Work out the finished part from the listing and answer in its coordinate system (mm). A direction names the side the tool comes from. Round coordinates to 2 decimals unless told otherwise and drop trailing zeros. Order: outer loops, then holes, each group sorted by start corner. A loop starts at its lowest first (then second) coordinate and runs counter-clockwise, first axis right, second up. Notation, with made-up numbers: (24.5, 38) - (68.5, 38) arc R10 ccw to (68.5, 53) - close; hole circle Ø7 at (35, 72.5). An arc over 180 degrees is marked (long way). Put each result on its own line as item: value.
```python
from build123d import *

# Parameters (mm, degrees)
BOSS_EXTRUDE1_DEPTH        = 4
BOSS_EXTRUDE2_REACH        = 34.985
F_2_CLEARANCE_HOLE1_D      = 2.5
F_12_CLEARANCE_HOLE1_D     = 6
F_4_CLEARANCE_HOLE1_REACH  = 43.113
F_4_CLEARANCE_HOLE1_BORE_R = 1.65
SKETCH9_W                  = 1.65
SKETCH9_H                  = 32
FILLET1_R                  = 2


with BuildPart() as part:
    # Sketch1 → Boss-Extrude1 (new body)
    with BuildSketch(Plane(origin=(0, 0, 12), x_dir=(-1, 0, 0), z_dir=(0, 0, -1))):
        with BuildLine():
            Line((-17.88854382, -16), (17.88854382, -16))
            ThreePointArc((17.88854382, -16), (24, 0), (17.88854382, 16))
            Line((17.88854382, 16), (-17.88854382, 16))
            ThreePointArc((-17.88854382, 16), (-24, 0), (-17.88854382, -16))
        make_face()
    extrude(amount=-BOSS_EXTRUDE1_DEPTH)

    # Sketch3 → Boss-Extrude2 (add, up to next)
    with BuildSketch(Plane(origin=(0, 0, 0), x_dir=(-1, 0, 0), z_dir=(0, 0, -1)), mode=Mode.PRIVATE) as boss_extrude2_sk1:
        with BuildLine():
            ThreePointArc((-15.821428571, 2.383778085), (-11, 0), (-15.821428571, -2.383778085))
            ThreePointArc((-15.821428571, -2.383778085), (0, -16), (15.821428571, -2.383778085))
            ThreePointArc((15.821428571, -2.383778085), (11, 0), (15.821428571, 2.383778085))
            ThreePointArc((15.821428571, 2.383778085), (0, 16), (-15.821428571, 2.383778085))
        make_face()
    boss_extrude2_tool1 = extrude(boss_extrude2_sk1.sketch, amount=-BOSS_EXTRUDE2_REACH, mode=Mode.PRIVATE) - part.part
    add(boss_extrude2_tool1.solids().sort_by_distance((0, 0, 0))[0])

    # #2 Clearance Hole1 (through all)
    with Locations(Plane(origin=(0, 0, 12), x_dir=(-1, 0, 0), z_dir=(0, 0, -1))):
        with Locations((21, 0), (-21, 0), (-14, 0), (14, 0)):
            Hole(F_2_CLEARANCE_HOLE1_D / 2)

    # #12 Clearance Hole1 (through all)
    with Locations(Plane(origin=(0, 0, 0), x_dir=(-1, 0, 0), z_dir=(0, 0, -1))):
        with Locations((0, 0)):
            Hole(F_12_CLEARANCE_HOLE1_D / 2)

    # #4 Clearance Hole1 bore (on position points) → #4 Clearance Hole1 (cut, up to next)
    with BuildSketch(Plane(origin=(0, 16, 9.5), x_dir=(1, 0, 0), z_dir=(0, 1, 0)), mode=Mode.PRIVATE) as f_4_clearance_hole1_sk1:
        Circle(F_4_CLEARANCE_HOLE1_BORE_R)
    f_4_clearance_hole1_tool1 = extrude(f_4_clearance_hole1_sk1.sketch, amount=-F_4_CLEARANCE_HOLE1_REACH, mode=Mode.PRIVATE) & part.part
    add(f_4_clearance_hole1_tool1.solids().sort_by_distance((0, 16, 9.5))[0], mode=Mode.SUBTRACT)

    # Sketch9 → #4 Clearance Hole2 (revolve, cut)
    with BuildSketch(Plane(origin=(0, -2.505493963, 3.5), x_dir=(0, 0, 1), z_dir=(1, 0, 0))):
        with Locations((0.825, 16)):
            Rectangle(SKETCH9_W, SKETCH9_H)
    revolve(axis=Axis((0, 3.844506037, 3.5), (0, -1, 0)), mode=Mode.SUBTRACT)

    # Fillet1
    fillet1_edges = [part.edges().sort_by_distance(p)[0] for p in [
        (15.821428571, -2.383778085, 6),
        (-15.821428571, -2.383778085, 6),
        (-15.821428571, 2.383778085, 6),
        (15.821428571, 2.383778085, 6),
    ]]
    fillet(fillet1_edges, radius=FILLET1_R)


solid = part.part
```
1) A cutting plane is placed at B-B on x = -20.5. Write down the section's boundary in (y, z).
Findings below:
outline: (-12.48, 12) - (-1.15, 12) - (-1.15, 16) - (-12.48, 16) - close; (1.15, 12) - (12.48, 12) - (12.48, 16) - (1.15, 16) - close
2) A cutting plane is placed at A-A on y = 0. Write down the section's boundary in (x, z), then the cut area to 3 significant figures.
Findings below:
outline: (-24, 12) - (-22.25, 12) - (-22.25, 16) - (-24, 16) - close; (-19.75, 12) - (-15.25, 12) - (-15.25, 16) - (-19.75, 16) - close; (-12.75, 12) - (-11, 12) - (-11, 0) - (-3, 0) - (-3, 16) - (-12.75, 16) - close; (3, 0) - (11, 0) - (11, 12) - (12.75, 12) - (12.75, 16) - (3, 16) - close; (15.25, 12) - (19.75, 12) - (19.75, 16) - (15.25, 16) - close; (22.25, 12) - (24, 12) - (24, 16) - (22.25, 16) - close
area: 320 mm2
3) A cutting plane is placed at D-D on y = -7. Write down the section's boundary in (x, z).
Findings below:
outline: (-22.96, 12) - (-14.39, 12) - (-14.39, 0) - (14.39, 0) - (14.39, 12) - (22.96, 12) - (22.96, 16) - (-22.96, 16) - close; hole circle Ø3.3 at (0, 3.5)
4) For a pull along Z with two mould halves and no side action, classify faces 1 (the cylindrical face through (-24, 0, 14)), 2 (the cylindrical face through (0.632, -9.349, 5.024)), 3 (the cylindrical face through (-0.4, 9.3, 11.1)), 4 (the flat face through (-17, 0, 12)) as pulls with the +Z half, pulls with the -Z half, needs draft (parallel to the pull), parting line crosses it, or undercut.
Findings below:
face 1: needs draft
face 2: undercut
face 3: undercut
face 4: pulls with the -Z half
5) Given pin 1 Ø3 at (y, z) = (-6.5, 2) entering from -X; pin 2 Ø2.5 at (x, z) = (0, 9.5) entering from +Y; pin 3 Ø6 at (y, z) = (-11.5, 2.5) entering from -X, each flat-ended and moving along its own axis, determine where each tip first touches the part or whether it passes through.
Findings below:
pin 1: stops at x = -15.11
pin 2: stops at y = -2.73
pin 3: stops at x = -13.56
6) A cutting plane is placed at C-C on x = 8. Write down the section's boundary in (y, z), then the cut area to 3 significant figures.
Findings below:
outline: (-16, 12) - (-13.86, 12) - (-13.86, 0) - (13.86, 0) - (13.86, 12) - (16, 12) - (16, 16) - (-16, 16) - close
area: 461 mm2
7) For faces 5 (the flat face through (18, 0, 12)), 6 (the cylindrical face through (0, 16, 6)), 7 (the cylindrical face through (0, -16, 6)), determine the directions among +Z, -Z, +X, -X, +Y, -Y from which every point of the face is accessible in a straight line to the end or side of a thin tool.
Findings below:
face 5: -Z, +X
face 6: -Z, +Y
face 7: -Z, -Y
8) Straight lines are drawn through the part: L1, parallel to Y at x = 0, z = 13; L2, parallel to Z at x = 0, y = 6.75; L3, parallel to Z at x = 0, y = -6. For each, find the intervals that lie inside material, in ascending order. Write a range as from..to.
Findings below:
L1: y = -16..-3, 3..16
L2: z = 0..7.85, 11.15..16
L3: z = 0..1.85, 5.15..16
